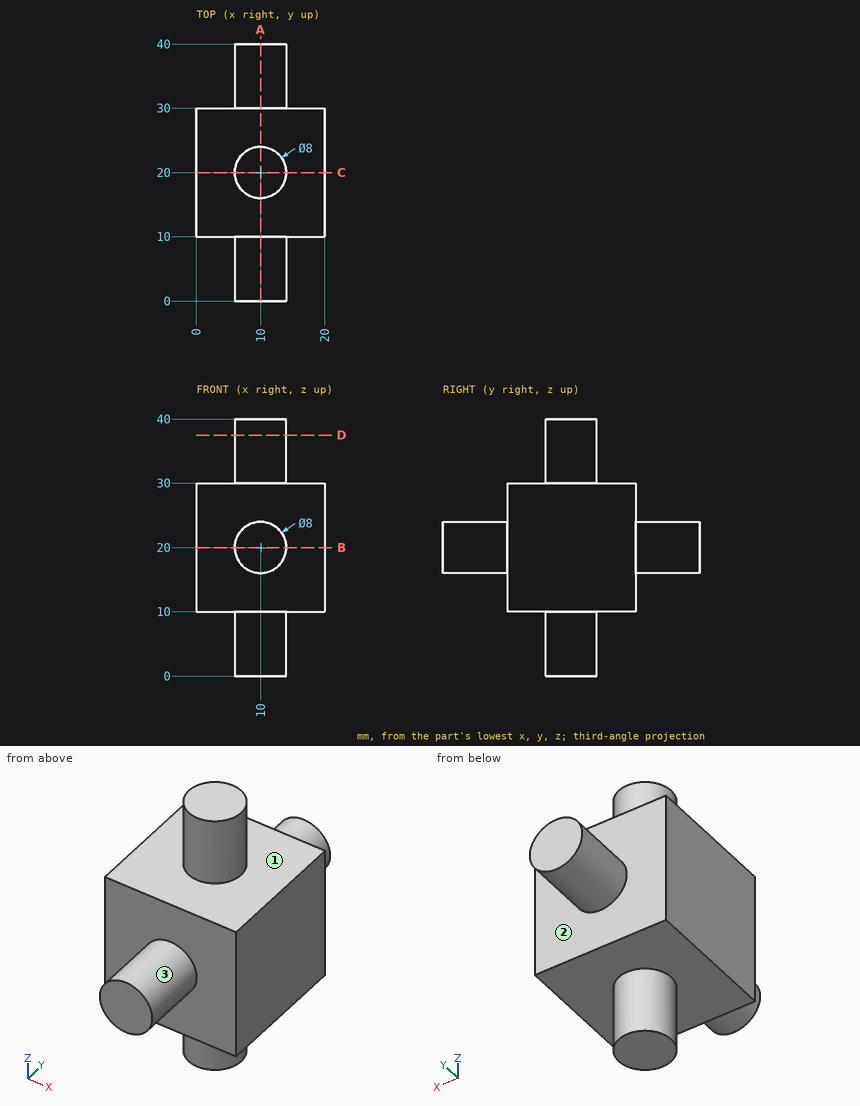
Answer from the drawing. Dimensions are ordinates in mm from the lowest x, y and z of the part. A direction names the side the tool comes from. Give positions to 0.01 mm unless a question says otherwise; leave off trailing zeros. Loops run counter-clockwise (first coordinate to the right, second up) from the corner with the lowest first, then second, coordinate; pieces in that order, holes last. Notation, with made-up numbers: (-8.75, 2) - (44.25, 2) arc R21 ccw to (44.25, 22) - close; hole circle Ø3 at (-34.75, 71). An arc over 180 degrees is marked (long way). Answer as CSV lines item,"result". Start each with the question number.
Item 1: Each of these flat-tipped pins is pushed along its axis until it touches: pin 1 (8 mm diameter, centred on x = 6.5, z = 29.5, fed in from -Y); pin 2 (1.5 mm diameter, centred on x = 7, y = 24.5, fed in from -Z); pin 3 (1 mm diameter, centred on x = 13.5, y = 14, fed in from +Z). Where does it stop, or does it pass through?
Item 2: A cutting plane is placed at A-A on x = 10. Determine the outline of the cut face in (y, z), then the cut area to 3 significant figures.
Item 3: A cutting plane is placed at D-D on z = 37.5. Determine the outline of the cut face in (x, y), then the cut area to 3 significant figures.
Item 4: Find the intervals of material crossed by line 1 (Z direction, x = 18.75, y = 14); line 2 (Z direction, x = 11.25, y = 33), in increasing order. Write a range as from..to.
Item 5: A cutting plane is placed at B-B on z = 20. Determine the outline of the cut face in (x, y), then the cut area to 3 significant figures.
Item 6: For the marked faces 1, 2 and 3, determine the directions among +Z, -Z, +X, -X, +Y, -Y from which every point of the face is accessible in a straight line to the end or side of a thin tool.
Found:
1,pin 1,"stops at y = 10"
1,pin 2,"stops at z = 10"
1,pin 3,"stops at z = 30"
2,outline,"(0, 16) - (10, 16) - (10, 10) - (16, 10) - (16, 0) - (24, 0) - (24, 10) - (30, 10) - (30, 16) - (40, 16) - (40, 24) - (30, 24) - (30, 30) - (24, 30) - (24, 40) - (16, 40) - (16, 30) - (10, 30) - (10, 24) - (0, 24) - close"
2,area,"720 mm^2"
3,outline,"circle Ø8 at (10, 20)"
3,area,"50.3 mm^2"
4,line 1,"z = 10..30"
4,line 2,"z = 16.2..23.8"
5,outline,"(0, 10) - (6, 10) - (6, 0) - (14, 0) - (14, 10) - (20, 10) - (20, 30) - (14, 30) - (14, 40) - (6, 40) - (6, 30) - (0, 30) - close"
5,area,"560 mm^2"
6,face 1,"+Z"
6,face 2,"+Y"
6,face 3,"-Y"
